Source: CAD feature listing. Evaluate the final solid. Frame: model axes, mm. A direction names the side the tool comes from. Give positions to 0.01 mm unless a question says otherwise; leave off trailing zeros. Write each loop counter-clockwise with the first axis right and the second up, starting at its lowest first coordinate (ties: lowest second). Pieces come first, ordered by that corner, then holes. Notation, with made-up numbers: (15.5, 58) -> (40.5, 58) arc R6 cw to (40.5, 68) -> close; hole circle Ø10 at (3.25, -34). An arc over 180 degrees is marked (long way). Use a Markdown table: item, result. Add a question column.
```python
from build123d import *

# Parameters (mm, degrees)
SKETCH1_R           = 1.5
BOSS_EXTRUDE1_DEPTH = 3


with BuildPart() as part:
    # Sketch1 → Boss-Extrude1 (new body)
    with BuildSketch(Plane(origin=(0, 0, 0), x_dir=(1, 0, 0), z_dir=(0, 1, 0))):
        Polygon((0, 9), (0, 0), (7.5, 0), (7.5, 1.5), (9.5, 1.5), (9.5, 0), (40, 0), (40, 2), (42, 2), (42, 0), (52, 0), (52, 35), (42, 35), (42, 33), (40, 33), (40, 35), (9.5, 35), (9.5, 33), (7.5, 33), (7.5, 35), (0, 35), (0, 21), (9.5, 21), (9.5, 22), (40, 22), (40, 8), (9.5, 8), (9.5, 9), align=None)
        with Locations(Location((48, 5, 0), (0, 0, 270))):
            Circle(SKETCH1_R, mode=Mode.SUBTRACT)
        with Locations(Location((48, 15, 0), (0, 0, 270))):
            Circle(SKETCH1_R, mode=Mode.SUBTRACT)
        with Locations(Location((4, 30, 0), (0, 0, 270))):
            Circle(SKETCH1_R, mode=Mode.SUBTRACT)
        with Locations(Location((19, 30, 0), (0, 0, 270))):
            Circle(SKETCH1_R, mode=Mode.SUBTRACT)
        with Locations(Location((29, 30, 0), (0, 0, 270))):
            Circle(SKETCH1_R, mode=Mode.SUBTRACT)
        with Locations(Location((48, 30, 0), (0, 0, 270))):
            Circle(SKETCH1_R, mode=Mode.SUBTRACT)
    extrude(amount=BOSS_EXTRUDE1_DEPTH)


solid = part.part
```
(1) Cut plane D-D on z = -15. Return the cut outline in (x, y).
(2) Cut plane A-A on x = 48. Return the cut outline in (y, z), then the cut area to 3 significant figures.
(3) Material intervals for L1, parallel to X at y = 1.1, z = -30; L2, parallel to Z at x = 39, y = 1.3; L3, parallel to Z at x = 5, y = 1.45, sorted ascending.
(4) First-contact query: pin 1 Ø6 at (x, z) = (36, -14) entering from -Y; pin 2 Ø0.6 at (x, y) = (8.5, 2) entering from -Z. Flat tips, straight axial feed; report the tip coordinate or a pass-through.
(5) Mould query, pull axis X, two halves, no side actions, for faces 5 (the flat face through (4, 1, 0)), 6 (the flat face through (0, 1, -5)), 7 (the flat face through (7.5, 1, -1)). Classes: +X half, -X half, draft (parallel to the pull), parting line (faces both ways), or undercut.
(6) Cut plane B-B on z = -30. Return the cut outline in (x, y), then the cut area to 3 significant figures.
(7) Access query for faces 1 (the flat face through (5, 1, -21)), 2 (the flat face through (40, 1, -34)), 3 (the flat face through (42, 1, -1)), 4 (the flat face through (9.5, 1.5, -21.5)). Directions: +Z, -Z, +X, -X, +Y, -Y. A direction counts if a zero-diameter tool reaches every point of the face in a straight line with its end or side. Return the directions, or none.
(8) Cut plane C-C on x = 29. Return the cut outline in (y, z).
Output:
| question | item | result |
|---|---|---|
| 1 | outline | (40, 0) -> (46.5, 0) -> (46.5, 3) -> (40, 3) -> close; (49.5, 0) -> (52, 0) -> (52, 3) -> (49.5, 3) -> close |
| 2 | outline | (0, -35) -> (3, -35) -> (3, -31.5) -> (0, -31.5) -> close; (0, -28.5) -> (3, -28.5) -> (3, -16.5) -> (0, -16.5) -> close; (0, -13.5) -> (3, -13.5) -> (3, -6.5) -> (0, -6.5) -> close; (0, -3.5) -> (3, -3.5) -> (3, 0) -> (0, 0) -> close |
| 2 | area | 78.0 mm^2 |
| 3 | L1 | 0 to 2.5, 5.5 to 17.5, 20.5 to 27.5, 30.5 to 46.5, 49.5 to 52 |
| 3 | L2 | -35 to -22, -8 to 0 |
| 3 | L3 | -35 to -31.12, -28.88 to -21, -9 to 0 |
| 4 | pin 1 | through |
| 4 | pin 2 | z = -33 |
| 5 | face 5 | draft |
| 5 | face 6 | -X half |
| 5 | face 7 | undercut |
| 6 | outline | (0, 0) -> (2.5, 0) -> (2.5, 3) -> (0, 3) -> close; (5.5, 0) -> (17.5, 0) -> (17.5, 3) -> (5.5, 3) -> close; (20.5, 0) -> (27.5, 0) -> (27.5, 3) -> (20.5, 3) -> close; (30.5, 0) -> (46.5, 0) -> (46.5, 3) -> (30.5, 3) -> close; (49.5, 0) -> (52, 0) -> (52, 3) -> (49.5, 3) -> close |
| 6 | area | 120 mm^2 |
| 7 | face 1 | -X, +Y, -Y |
| 7 | face 2 | -Z, +Y, -Y |
| 7 | face 3 | +Z, +Y, -Y |
| 7 | face 4 | +Y, -Y |
| 8 | outline | (0, -35) -> (3, -35) -> (3, -31.5) -> (0, -31.5) -> close; (0, -28.5) -> (3, -28.5) -> (3, -22) -> (0, -22) -> close; (0, -8) -> (3, -8) -> (3, 0) -> (0, 0) -> close |
